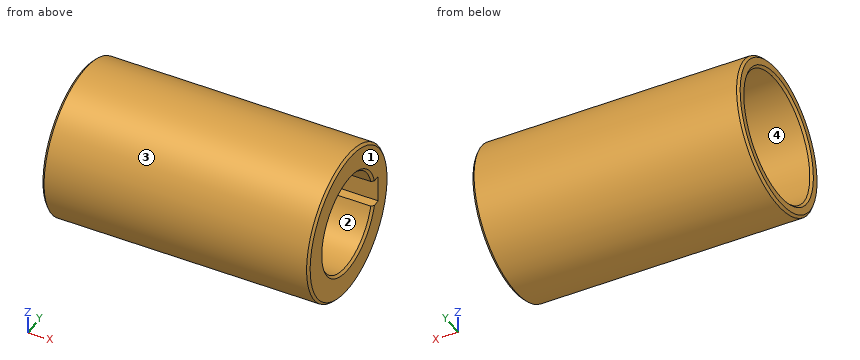
```python
from build123d import *

# Parameters (mm, degrees)
CHAMFER1_SIZE      = 1
SKETCH2_W          = 12
SKETCH2_H          = 8.3
CUT_EXTRUDE1_DEPTH = 100


with BuildPart() as part:
    # Sketch1 → Revolve1 (revolve)
    with BuildSketch(Plane.XY, mode=Mode.PRIVATE) as revolve1_sk:
        Polygon((0, 27.5), (0, 32.5), (115, 32.5), (115, 21), (63, 21), (63, 27.5), align=None)
    revolve(revolve1_sk.sketch.rotate(Axis((0, 0, 0), (1, 0, 0)), 90), axis=Axis((0, 0, 0), (1, 0, 0)))

    # Chamfer1
    chamfer1_edges = [part.edges().sort_by_distance(p)[0] for p in [
        (115, 0, -21),
        (115, 0, -32.5),
        (0, 0, -32.5),
        (0, 0, -27.5),
    ]]
    chamfer(chamfer1_edges, length=CHAMFER1_SIZE)

    # Sketch2 → Cut-Extrude1 (cut)
    with BuildSketch(Plane(origin=(115, 0, 0), x_dir=(0, 0, -1), z_dir=(1, 0, 0))):
        with Locations((0, 20.15)):
            Rectangle(SKETCH2_W, SKETCH2_H)
    extrude(amount=-CUT_EXTRUDE1_DEPTH, mode=Mode.SUBTRACT)


solid = part.part
```
Geometry: final body of the model. Coordinates: model frame, mm. Face numbers are marked on the shaded views. Give positions to 0.01 mm unless a question says otherwise; leave off trailing zeros. Loops run counter-clockwise (first coordinate to the right, second up) from the corner with the lowest first, then second, coordinate; pieces in that order, holes last. Notation, with made-up numbers: (22.25, 64.5) -> (34.25, 64.5) arc R34 ccw to (34.25, 102.5) -> close; hole circle Ø3 at (41, 71). An arc over 180 degrees is marked (long way). Use one line per item in the form item = value.
Item 1: Section query C-C on x = 27.5. Output: boundary loops of the cut face in (y, z).
A:
outline = circle Ø65 at (0, 0); hole circle Ø55 at (0, 0)
Item 2: Section query A-A on y = 0. Output: boundary loops of the cut face in (x, z).
A:
outline = (0, -31.5) -> (1, -32.5) -> (114, -32.5) -> (115, -31.5) -> (115, -22) -> (114, -21) -> (63, -21) -> (63, -27.5) -> (1, -27.5) -> (0, -28.5) -> close; (0, 28.5) -> (1, 27.5) -> (63, 27.5) -> (63, 21) -> (114, 21) -> (115, 22) -> (115, 31.5) -> (114, 32.5) -> (1, 32.5) -> (0, 31.5) -> close
Item 3: Draft query along Y for the marked faces 1, 2, 3 and 4. Return one class per face: pulls with the +Y half, pulls with the -Y half, needs draft (parallel to the pull), parting line crosses it, or undercut.
A:
face_1 = needs draft
face_2 = undercut
face_3 = parting line crosses it
face_4 = undercut
Item 4: Pin query (flat end, axial travel): P1, Ø1, axis at x = 51.5, z = -1.5, coming from the +Y side; P2, Ø12, axis at x = 14, y = -23, coming from the -Z side; P3, Ø5, axis at x = 69.5, z = 16.5, coming from the +Y side. Return the tip coordinate at first contact, or that it passes through.
A:
P1 = 32.48
P2 = -27.7
P3 = 29.33
Item 5: Line query: probe 1 along Y at (x, z) = (41, 0); probe 2 along Z at (x, y) = (5, -1); probe 3 along Y at (x, z) = (96.5, 0). Output: solid intervals per line, ascending.
A:
probe_1 = -32.5 to -27.5, 27.5 to 32.5
probe_2 = -32.48 to -27.48, 27.48 to 32.48
probe_3 = -32.5 to -21, 24.3 to 32.5
Item 6: Section query B-B on z = 0. Output: boundary loops of the cut face in (x, y), and give its area (3 significant figures).
A:
outline = (0, -31.5) -> (1, -32.5) -> (114, -32.5) -> (115, -31.5) -> (115, -22) -> (114, -21) -> (63, -21) -> (63, -27.5) -> (1, -27.5) -> (0, -28.5) -> close; (0, 28.5) -> (1, 27.5) -> (63, 27.5) -> (63, 24.3) -> (115, 24.3) -> (115, 31.5) -> (114, 32.5) -> (1, 32.5) -> (0, 31.5) -> close
area = 1,650 mm^2
Item 7: Section query D-D on x = 107. Output: boundary loops of the cut face in (y, z).
A:
outline = circle Ø65 at (0, 0); hole (20.12, -6) -> (24.3, -6) -> (24.3, 6) -> (20.12, 6) arc R21 ccw (long way) to start
